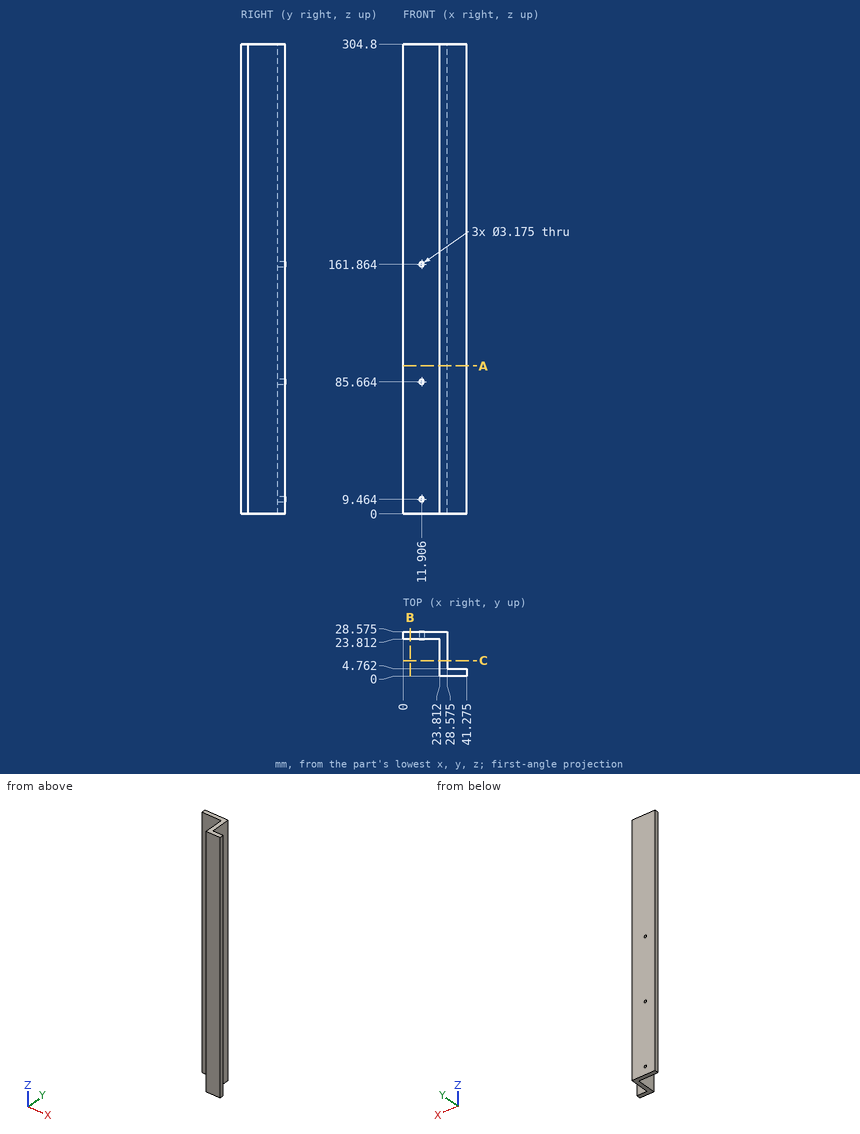
Can you work these out from the drawing? Everything is in mm from the part's minimum corner. Give positions to 0.01 mm unless a question says otherwise; leave off trailing zeros. Write each loop counter-clockwise with the first axis right and the second up, starting at its lowest first coordinate (ties: lowest second). Pieces come first, ordered by that corner, then holes. Notation, with made-up numbers: M 86,8.5 L 143,8.5 A32 ccw 143,40.5 Z; hole C -24,19 d11. An arc over 180 degrees is marked long. Answer in a Markdown table with one row per item. Add a question column.
Item 1: Imagine slicing it at B-B, the plane x = 4.5. Write out the boundary of the cut face in (y, z) (1 decimal).
Item 2: Imagine slicing it at A-A, the plane z = 96. Write out the boundary of the cut face in (x, y) (1 decimal).
Item 3: For pin 1 Ø5 at (y, z) = (6.5, 246) entering from -X; pin 2 Ø12 at (y, z) = (17, 220.5) entering from +X (1 decimal); pin 3 Ø4 at (x, z) = (11.5, 68) entering from -Y, each with a flat end and sliding along its axis, tell me the tip position at first contact or that it passes through.
Item 4: Please list where these lines run through material, in increasing order: L1, parallel to Y at x = 19.5, z = 152 (1 decimal); L2, parallel to X at y = 3.5, z = 94.5 (1 decimal).
Evaluation:
| question | item | result |
|---|---|---|
| 1 | outline | M 23.8,0 L 28.6,0 L 28.6,304.8 L 23.8,304.8 Z |
| 2 | outline | M 0,23.8 L 23.8,23.8 L 23.8,0 L 41.3,0 L 41.3,4.8 L 28.6,4.8 L 28.6,28.6 L 0,28.6 Z |
| 3 | pin 1 | stops at x = 23.81 |
| 3 | pin 2 | stops at x = 28.6 |
| 3 | pin 3 | stops at y = 23.81 |
| 4 | L1 | y = 23.8 to 28.6 |
| 4 | L2 | x = 23.8 to 41.3 |
